from build123d import *

# Parameters (mm, degrees)
F0_W     = 120.65
F0_H     = 80
F1_DEPTH = 25.4
F3_DEPTH = 19.05
F4_R     = 20.64
F5_DEPTH = 16
F7_DEPTH = 19.05
F8_R     = 14.9987
F9_DEPTH = 25.401


with BuildPart() as f1:
    # F0 (on Top) → F1 (new body)
    with BuildSketch(Plane.XY):
        Rectangle(F0_W, F0_H)
    extrude(amount=F1_DEPTH)

    # F2 (on face) → F3 (cut)
    with BuildSketch(Plane.YZ.offset(60.325)):
        Polygon((21.952974, 28.64855), (3.992462, 10.688038), (39.347801, -24.667301), (57.308314, -6.706789), align=None)
    extrude(amount=-F3_DEPTH, mode=Mode.SUBTRACT)

    # F4 (on face) → F5 (cut)
    with BuildSketch(Plane.XY.offset(25.4)):
        with Locations((0, -5)):
            Circle(F4_R)
    extrude(amount=-F5_DEPTH, mode=Mode.SUBTRACT)

    # F6 (on face) → F7 (cut)
    with BuildSketch(Plane(origin=(-60.325, 0, 0), x_dir=(0, -1, 0), z_dir=(-1, 0, 0))):
        Polygon((-21.943312, 28.653912), (-57.307561, -6.710336), (-39.347049, -24.670849), (-3.9828, 10.6934), align=None)
    extrude(amount=-F7_DEPTH, mode=Mode.SUBTRACT)

    # F8 (on face) → F9 (cut, through all)
    with BuildSketch(Plane.XY.offset(25.4)):
        with Locations((0, -5)):
            Circle(F8_R)
    extrude(amount=-F9_DEPTH, mode=Mode.SUBTRACT)


solid = f1.part
The listing builds one solid part. Answer for the finished solid, in the listing's coordinates (mm). A direction names the side the tool comes from. Give positions to 0.01 mm unless a question says otherwise; leave off trailing zeros. Order: outer loops, then holes, each group sorted by start corner. A loop starts at its lowest first (then second) coordinate and runs counter-clockwise, first axis right, second up. Notation, with made-up numbers: (83, -6) -> (109, -6) arc R37 cw to (109, 32) -> close; hole circle Ø10 at (51.25, 70.25). An arc over 180 degrees is marked (long way). Put each result on its own line as item: value.
Item 1: For faces 1 (the face through (-50.9, 32.5, 18.1)), 2 (the face through (-1, 40, 13)), 3 (the face through (-41.275, 22, 10)), 4 (the face through (-16.38, -17.56, 17.51)), 5 (the face through (41.275, 22, 10)), determine the directions among +Z, -Z, +X, -X, +Y, -Y from which every point of the face is accessible in a straight line to the end or side of a thin tool.
Established:
face 1: -Z, -X
face 2: +Z, -Z, +X, -X, +Y
face 3: -X
face 4: +Z
face 5: +X
Item 2: For a pull along X with two mould halves and no side action, classify faces 6 (the face through (-14.984, -4.341, 4.766)), 7 (the face through (60.325, -18, 13)), 8 (the face through (50.9, 32.7, 17.9)), 9 (the face through (14, 1, 9.4)) as released by +X, released by -X, zero draft, split by the parting line, or undercut.
Established:
face 6: undercut
face 7: released by +X
face 8: zero draft
face 9: undercut
Item 3: Straight lines are drawn through the part: line 1 (Y direction, x = 0, z = 14); line 2 (Y direction, x = 0, z = 2.5); line 3 (X direction, y = 18, z = 15.75) (3 decimals). For each, find the intervals that lie inside material, in ascending order.
Established:
line 1: y = -40 to -25.64, 15.64 to 40
line 2: y = -40 to -20, 10 to 40
line 3: x = -41.275 to 41.275
Item 4: A cutting plane is placed at C-C on z = 19.25. Give the vertices of the cut face in (x, y) (3 decimals).
Established:
outline: (-60.325, -40) -> (60.325, -40) -> (60.325, 12.554) -> (41.275, 12.554) -> (41.275, 31.352) -> (60.325, 31.352) -> (60.325, 40) -> (-60.325, 40) -> (-60.325, 31.347) -> (-41.275, 31.347) -> (-41.275, 12.539) -> (-60.325, 12.539) -> close; hole circle Ø41.28 at (0, -5)
Item 5: A cutting plane is placed at D-D on x = 0. Give the vertices of the cut face in (y, z).
Established:
outline: (-40, 0) -> (-20, 0) -> (-20, 9.4) -> (-25.64, 9.4) -> (-25.64, 25.4) -> (-40, 25.4) -> close; (10, 0) -> (40, 0) -> (40, 25.4) -> (15.64, 25.4) -> (15.64, 9.4) -> (10, 9.4) -> close
Item 6: A cutting plane is placed at A-A on y = -5. Give the vertices of the cut face in (x, z) (3 decimals), plus the area to 3 significant figures.
Established:
outline: (-60.325, 0) -> (-14.999, 0) -> (-14.999, 9.4) -> (-20.64, 9.4) -> (-20.64, 25.4) -> (-60.325, 25.4) -> close; (14.999, 0) -> (60.325, 0) -> (60.325, 25.4) -> (20.64, 25.4) -> (20.64, 9.4) -> (14.999, 9.4) -> close
area: 2,120 mm^2
Item 7: A cutting plane is placed at B-B on x = 51. Give the vertices of the cut face in (y, z), plus the area to 3 significant figures.
Established:
outline: (-40, 0) -> (14.68, 0) -> (3.99, 10.69) -> (18.7, 25.4) -> (-40, 25.4) -> close; (25.2, 25.4) -> (40, 10.6) -> (40, 25.4) -> close
area: 1,390 mm^2
